Model file for the job. Use its own axes, mm. A direction names the side the tool comes from. Coordinates: 2 decimals unless noted, no trailing zeros. Order: outer loops, then holes, each group sorted by start corner. A loop starts at its lowest first (then second) coordinate and runs counter-clockwise, first axis right, second up. Notation, with made-up numbers: M 44,70.25 L 67,70.25 A12 ccw 67,74.25 Z; hole C 7,12.5 d4. An arc over 180 degrees is marked long. Return JSON: item names as keys, results as strings.
```python
from build123d import *

# Parameters (mm, degrees)
CUT_EXTRUDE1_DEPTH = 25


with BuildPart() as part:
    # Sketch1 → Revolve1 (revolve)
    with BuildSketch(Plane.XY, mode=Mode.PRIVATE) as revolve1_sk:
        with BuildLine():
            Line((0, -150), (-5.5, -150))
            Line((-5.5, -150), (-5.5, -34.1))
            Line((-5.5, -34.1), (-17.75, -34.1))
            Line((-17.75, -34.1), (-17.75, -25.3))
            Line((-17.75, -25.3), (-25.75, -25.3))
            Line((-25.75, -25.3), (-25.75, -23.8))
            Line((-25.75, -23.8), (-17, -20))
            Line((-17, -20), (-17, -18))
            Line((-17, -18), (-11.624443868, 2.97864143))
            ThreePointArc((-11.624443868, 2.97864143), (-7.357183661, 9.480076402), (0, 12))
            Line((0, 12), (0, -150))
        make_face()
    revolve(revolve1_sk.sketch.rotate(Axis((0, -150, 0), (0, 1, 0)), 180), axis=Axis((0, -150, 0), (0, 1, 0)))

    # Sketch2 → Cut-Extrude1 (cut, symmetric)
    with BuildSketch(Plane(origin=(0, 0, 0), x_dir=(0, 0, -1), z_dir=(1, 0, 0))):
        with BuildLine():
            Line((-4.2, 12.434179723), (-4.2, -13))
            ThreePointArc((-4.2, -13), (-5.664466094, -16.535533906), (-9.2, -18))
            Line((-9.2, -18), (-21.107877624, -18))
            Line((-21.107877624, -18), (-21.107877624, 12.434179723))
            Line((-21.107877624, 12.434179723), (-4.2, 12.434179723))
        make_face()
        with BuildLine():
            Line((21.107877624, 12.434179723), (4.2, 12.434179723))
            Line((4.2, 12.434179723), (4.2, -13))
            ThreePointArc((4.2, -13), (5.664466094, -16.535533906), (9.2, -18))
            Line((9.2, -18), (21.107877624, -18))
            Line((21.107877624, -18), (21.107877624, 12.434179723))
        make_face()
    extrude(amount=CUT_EXTRUDE1_DEPTH, both=True, mode=Mode.SUBTRACT)

    # Sketch3 → Cut-Revolve1 (revolve, cut)
    with BuildSketch(Plane.XY):
        with BuildLine():
            Line((0, -6.5), (0, 6.5))
            ThreePointArc((0, 6.5), (-6.5, 0), (0, -6.5))
        make_face()
    revolve(axis=Axis((0, -6.5, 0), (0, 1, 0)), mode=Mode.SUBTRACT)


solid = part.part
```
Item 1: Saw through at B-B (x = 0). Write the cut outline in (y, z).
Check result:
{"outline": "M -150,-5.5 L -34.1,-5.5 L -34.1,-17.75 L -25.3,-17.75 L -25.3,-25.75 L -23.8,-25.75 L -20,-17 L -18,-17 L -18,-9.2 A5 cw -13,-4.2 L -4.96,-4.2 A6.5 cw -4.96,4.2 L -13,4.2 A5 cw -18,9.2 L -18,17 L -20,17 L -23.8,25.75 L -25.3,25.75 L -25.3,17.75 L -34.1,17.75 L -34.1,5.5 L -150,5.5 Z; M 4.96,-4.2 L 11.24,-4.2 A12 ccw 11.24,4.2 L 4.96,4.2 A6.5 cw Z"}
Item 2: Drop flat-ended pins along their axis: pin 1 Ø1 at (x, z) = (11, -18.5) entering from -Y; pin 2 Ø2 at (x, y) = (6, -115.5) entering from +Z; pin 3 Ø19.5 at (x, y) = (7, -3) entering from +Z; pin 4 Ø12 at (y, z) = (-77.5, 13) entering from +X. Give the stop position or say it passes through.
Check result:
{"pin 1": "stops at y = -25.3", "pin 2": "stops at z = 2.29", "pin 3": "stops at z = 4.2", "pin 4": "passes through"}
Item 3: 3-axis set-ups, long thin cutter, end or side, ignore diameter. For faces 1 (the cylindrical face through (-2.213, -18.986, -16.855)), 2 (the cylindrical face through (-3.848, -29.638, 17.328)), 3 (the flat face through (0, -6, -4.2)), 4 (the flat face through (0, -18, 12)): which of +Z, -Z, +X, -X, +Y, -Y reach the whole face in a straight line?
Check result:
{"face 1": "+Y", "face 2": "-Y", "face 3": "-Z, +X, -X, +Y", "face 4": "+Z, +X, -X, +Y"}
Item 4: Wall check: line 1 (Y direction, x = -1.5, z = -2.5); line 2 (Z direction, x = 0.5, y = -52); line 3 (Y direction, x = -1.5, z = -2). Give the ranges that are in metal, low to high.
Check result:
{"line 1": "y = -150 to -5.81, 5.81 to 11.64", "line 2": "z = -5.48 to 5.48", "line 3": "y = -150 to -6, 6 to 11.74"}
Item 5: Saw through at C-C (y = -133.5). Write the cut outline in (x, z).
Check result:
{"outline": "C 0,0 d11"}
Item 6: Saw through at A-A (z = 0). Write the cut outline in (x, y).
Check result:
{"outline": "M -25.75,-25.3 L -17.75,-25.3 L -17.75,-34.1 L -5.5,-34.1 L -5.5,-150 L 5.5,-150 L 5.5,-34.1 L 17.75,-34.1 L 17.75,-25.3 L 25.75,-25.3 L 25.75,-23.8 L 17,-20 L 17,-18 L 11.62,2.98 A12 ccw -11.62,2.98 L -17,-18 L -17,-20 L -25.75,-23.8 Z; hole C 0,0 d13"}
